For this review, take the finished solid that the model builds, in its own axes (mm). A direction names the side the tool comes from. Round coordinates to 2 decimals unless told otherwise and drop trailing zeros. Order: outer loops, then holes, each group sorted by start corner. A loop starts at its lowest first (then second) coordinate and runs counter-clockwise, first axis right, second up. Notation, with made-up numbers: M 21.5,73.25 L 79.5,73.25 A16 ccw 79.5,98.25 Z; hole C -32,-29 d5. An arc over 180 degrees is marked long. Answer in a Markdown table with one row per item. Add a question column.
```python
from build123d import *

# Parameters (mm, degrees)
F2_R     = 4.9
F3_DEPTH = 13
F2_R_2   = 12.25
F4_DEPTH = 1
F5_SIZE  = 2


with BuildPart() as f1:
    # F0 (on Front) → F1 (revolve)
    with BuildSketch(Plane.XZ):
        with BuildLine():
            Line((0, -19.3), (0, 0))
            Line((0, 0), (-68, 0))
            Line((-68, 0), (-68, -6.3))
            ThreePointArc((-68, -6.3), (-63.6066017178, -16.9066017178), (-53, -21.3))
            Line((-53, -21.3), (-42, -21.3))
            Line((-42, -21.3), (-42, -19.3))
            Line((-42, -19.3), (0, -19.3))
        make_face()
    revolve(axis=Axis((0, 0, -9.65), (0, 0, -1)))

    # F2 (on face) → F3 (join)
    with BuildSketch(Plane.XY):
        with Locations((-50, -10)):
            Circle(F2_R)
        with Locations((-25, -30)):
            Circle(F2_R)
        with Locations((0, -10)):
            Circle(F2_R)
        with Locations((25, -30)):
            Circle(F2_R)
        with Locations((50, -10)):
            Circle(F2_R)
    extrude(amount=F3_DEPTH)

    # F2 (on face) → F4 (join)
    with BuildSketch(Plane.XY):
        with Locations((-50, -10)):
            Circle(F2_R_2)
        with Locations((-50, -10)):
            Circle(F2_R, mode=Mode.SUBTRACT)
        with Locations((-25, -30)):
            Circle(F2_R_2)
        with Locations((-25, -30)):
            Circle(F2_R, mode=Mode.SUBTRACT)
        with Locations((0, -10)):
            Circle(F2_R_2)
        with Locations((0, -10)):
            Circle(F2_R, mode=Mode.SUBTRACT)
        with Locations((25, -30)):
            Circle(F2_R_2)
        with Locations((25, -30)):
            Circle(F2_R, mode=Mode.SUBTRACT)
        with Locations((50, -10)):
            Circle(F2_R_2)
        with Locations((50, -10)):
            Circle(F2_R, mode=Mode.SUBTRACT)
    extrude(amount=F4_DEPTH)

    # F5
    f5_edges = [f1.edges().sort_by_distance(p)[0] for p in [
        (-54.9, -10, 13),
        (-29.9, -30, 13),
        (-4.9, -10, 13),
        (20.1, -30, 13),
        (45.1, -10, 13),
    ]]
    chamfer(f5_edges, length=F5_SIZE)

    # F7 (on offset) → F8 (revolve, cut)
    with BuildSketch(Plane.XY.offset(2.5)):
        Polygon((-31, 0), (-25, 0), (-25, 35), (-25, 39), (-25, 48), (-35, 48), (-35, 39), (-38, 39), (-38, 35), (-31, 35), align=None)
    revolve(axis=Axis((-25, 17.5, 2.5), (0, 1, 0)), mode=Mode.SUBTRACT)

    # F7 (on offset) → F9 (revolve, cut)
    with BuildSketch(Plane.XY.offset(2.5)):
        Polygon((25, 35), (25, 0), (31, 0), (31, 35), (38, 35), (38, 39), (35, 39), (35, 48), (25, 48), (25, 39), align=None)
    revolve(axis=Axis((25, 17.5, 2.5), (0, 1, 0)), mode=Mode.SUBTRACT)


solid = f1.part
```
1. Consider section C-C on z = -16. Write out the cut boundary in (x, y).
2. Consider section A-A on z = 4.5. Write out the cut boundary in (x, y).
3. Clearance check with flat-ended pins moving along their axes: pin 1 Ø6 at (y, z) = (-18.5, -2) entering from -X; pin 2 Ø3 at (x, z) = (-29, -4.5) entering from -Y; pin 3 Ø11.5 at (x, z) = (22.5, -4.5) entering from -Y; pin 4 Ø3 at (x, z) = (6.5, 6.5) entering from +Y. State where each tip first meets the part, or that it passes through.
4. For faces 5 (the cylindrical face through (-40.06, 12.62, -20.29)), 6 (the flat face through (50, -10, 13)), 7 (the cylindrical face through (-13.316, -26.32, 0.493)), list the 3-axis set-ups (+Z, -Z, +X, -X, +Y, -Y) from which the entire face can be reached by the end or side of a thin tool; tool diameter is ignored.
5. The part is to be moulded in two halves that separate along Y. For faces 1 (the flat face through (-25, -30, 13)), 2 (the cylindrical face through (-36.556, 57.338, -3.194)), 3 (the flat face through (-25, 0, -1)), 4 (the cylindrical face through (25.2, 43.6, -7.5)), say which applies: pulls with the +Y half, pulls with the -Y half, needs draft (parallel to the pull), parting line crosses it, or undercut.
6. To check wall thickness, follow probe 1 along Z at (x, y) = (-4, 24); probe 2 along Z at (x, y) = (-38.5, -35); probe 3 along Y at (x, z) = (26, -7). State the ranges of each line that lie inside material, in increasing order. Write a range as [from, to].
7. Consider section B-B on x = 0. Write out the cut boundary in (y, z).
Solved:
| question | item | result |
|---|---|---|
| 1 | outline | C 0,0 d128.88 |
| 2 | outline | C -50,-10 d9.8; C -25,-30 d9.8; C 0,-10 d9.8; C 25,-30 d9.8; C 50,-10 d9.8 |
| 3 | pin 1 | stops at x = -66.21 |
| 3 | pin 2 | stops at y = -62.19 |
| 3 | pin 3 | stops at y = -65.9 |
| 3 | pin 4 | passes through |
| 4 | face 5 | -Z |
| 4 | face 6 | +Z, +X, -X, +Y, -Y |
| 4 | face 7 | +Z |
| 5 | face 1 | needs draft |
| 5 | face 2 | parting line crosses it |
| 5 | face 3 | undercut |
| 5 | face 4 | undercut |
| 6 | probe 1 | z = [-19.3, 0] |
| 6 | probe 2 | z = [-21.3, 0] |
| 6 | probe 3 | y = [-62.82, 35], [48, 62.82] |
| 7 | outline | M -68,-6.3 A15 ccw -53,-21.3 L -42,-21.3 L -42,-19.3 L 42,-19.3 L 42,-21.3 L 53,-21.3 A15 ccw 68,-6.3 L 68,0 L 2.25,0 L 2.25,1 L -5.1,1 L -5.1,11 L -7.1,13 L -12.9,13 L -14.9,11 L -14.9,1 L -22.25,1 L -22.25,0 L -68,0 Z |
